Part model, mm, in its own coordinate system. A direction names the side the tool comes from. Round coordinates to 2 decimals unless told otherwise and drop trailing zeros. Loops run counter-clockwise (first coordinate to the right, second up) from the corner with the lowest first, then second, coordinate; pieces in that order, holes last. Notation, with made-up numbers: (72, 65.25) - (89, 65.25) arc R11 cw to (89, 83.25) - close; hole circle Ø11 at (9, -19.5). An arc over 180 degrees is marked (long way). Write each question's results on one line, items separated by ' | '. Start each with the question number.
(1) Cut at B-B, the plane z = 5.5. List the corners of the cut face in (x, y).
(2) Drill centre lines: L1, parallel to Y at x = -20.5, z = 40.5; L2, parallel to Y at x = -155, z = 13; L3, parallel to Z at x = -43.5, y = 14. Where is each one in solid material? Low to high.
(3) Cut at A-A, the plane x = -118.5. List the corners of the cut face in (y, z).
(4) Flat gauge pins, fed straight in: P1, Ø4, axis at y = -4, z = 32, coming from the +X side; P2, Ø1, axis at x = -34, y = 15, coming from the -Z side; P3, Ø10, axis at x = 8.5, z = 37, coming from the +Y side. Where does each tip first touch, or does it go through?
(5) Mould opens along Y. For faces 1 (the face through (-86, -40, 23)), 2 (the face through (-72, 37, 25)), 3 (the face through (12, 38.3, 35)) say: released by +Y, released by -Y, zero draft, split by the parting line, or undercut.
(6) Tool access for faces 4 (the face through (-85, 38.3, 12)), 5 (the face through (12, -38.3, 35)), 6 (the face through (12, 1, 45.5)): list every direction of +Z, -Z, +X, -X, +Y, -Y with a clear straight run to the whole face (end or side of a thin tool).
(7) Cut at C-C, the plane y = -16.5. List the corners of the cut face in (x, z), then the cut area to 4 significant figures.
(8) Cut at D-D, the plane z = 29. List the corners of the cut face in (x, y).
from build123d import *

# Parameters (mm, degrees)
F1_DEPTH  = 43.5
F2_W      = 170
F2_H      = 80
F3_DEPTH  = 4
F5_DEPTH  = 25
F6_W      = 25
F6_H      = 2
F7_DEPTH  = 43.5
F9_DEPTH  = 25
F10_W     = 25
F10_H     = 0.3
F11_DEPTH = 18.5
F12_W     = 25
F12_H     = 2.3
F12_H_2   = 2
F13_DEPTH = 18.5
F15_DEPTH = 25


with BuildPart() as f1:
    # F0 (on Top) → F1 (new body)
    with BuildSketch(Plane.XY):
        Polygon((-166, 0), (-166, 36), (0, 36), (0, 40), (-170, 40), (-170, -40), (0, -40), (0, -36), (-166, -36), align=None)
    extrude(amount=F1_DEPTH)

    # F2 (on face) → F3 (join)
    with BuildSketch(Plane.XY.offset(43.5)):
        with Locations((-85, 0)):
            Rectangle(F2_W, F2_H)
    extrude(amount=F3_DEPTH)

    # F4 (on face) → F5 (cut)
    with BuildSketch(Plane.XY):
        Polygon((0, -36), (-166, -36), (-166, 0), (-166, 36), (0, 36), (0, 38), (-168, 38), (-168, -38), (0, -38), align=None)
    extrude(amount=F5_DEPTH, mode=Mode.SUBTRACT)

    # F6 (on face) → F7 (cut)
    with BuildSketch(Plane.XY):
        with Locations((-12.5, -37)):
            Rectangle(F6_W, F6_H)
        with Locations((-12.5, 37)):
            Rectangle(F6_W, F6_H)
    extrude(amount=F7_DEPTH, mode=Mode.SUBTRACT)

    # F8 (on face) → F9 (cut)
    with BuildSketch(Plane(origin=(0, 0, 0), x_dir=(1, 0, 0), z_dir=(0, 0, -1))):
        Polygon((-168, -38), (-168, 38), (0, 38), (0, 38.3), (-168.3, 38.3), (-168.3, -38.3), (0, -38.3), (0, -38), align=None)
    extrude(amount=-F9_DEPTH, mode=Mode.SUBTRACT)

    # F10 (on face) → F11 (cut)
    with BuildSketch(Plane(origin=(0, 0, 25), x_dir=(1, 0, 0), z_dir=(0, 0, -1))):
        with Locations((-12.5, 38.15)):
            Rectangle(F10_W, F10_H)
    extrude(amount=-F11_DEPTH, mode=Mode.SUBTRACT)

    # F12 (on face) → F13 (join)
    with BuildSketch(Plane(origin=(0, 0, 25), x_dir=(1, 0, 0), z_dir=(0, 0, -1))):
        with Locations((-12.5, 37.15)):
            Rectangle(F12_W, F12_H)
        with Locations((-12.5, -37)):
            Rectangle(F12_W, F12_H_2)
    extrude(amount=-F13_DEPTH)

    # F14 (on face) → F15 (join)
    with BuildSketch(Plane.YZ):
        Polygon((-36, 43.5), (36, 43.5), (36, 25), (38.3, 25), (38.3, 45.5), (-38.3, 45.5), (-38.3, 25), (-36, 25), align=None)
    extrude(amount=F15_DEPTH)


solid = f1.part
A:
1) outline: (-170, -40) - (0, -40) - (0, -38.3) - (-168.3, -38.3) - (-168.3, 38.3) - (0, 38.3) - (0, 40) - (-170, 40) - close
2) L1: -40 to -36, 36 to 40 | L2: -40 to -38.3, 38.3 to 40 | L3: 43.5 to 47.5
3) outline: (-40, 0) - (-38.3, 0) - (-38.3, 25) - (-36, 25) - (-36, 43.5) - (36, 43.5) - (36, 25) - (38.3, 25) - (38.3, 0) - (40, 0) - (40, 47.5) - (-40, 47.5) - close
4) P1: x = -166 | P2: z = 43.5 | P3: y = 38.3
5) face 1: released by -Y | face 2: undercut | face 3: released by +Y
6) face 4: -Z, +X | face 5: +Z, -Z, +X, -Y | face 6: +Z, +X, +Y, -Y
7) outline: (-170, 0) - (-168.3, 0) - (-168.3, 25) - (-166, 25) - (-166, 43.5) - (25, 43.5) - (25, 45.5) - (0, 45.5) - (0, 47.5) - (-170, 47.5) - close | area: 846.5 mm2
8) outline: (-170, -40) - (0, -40) - (0, -38.3) - (25, -38.3) - (25, -36) - (-166, -36) - (-166, 36) - (25, 36) - (25, 38.3) - (0, 38.3) - (0, 40) - (-170, 40) - close
